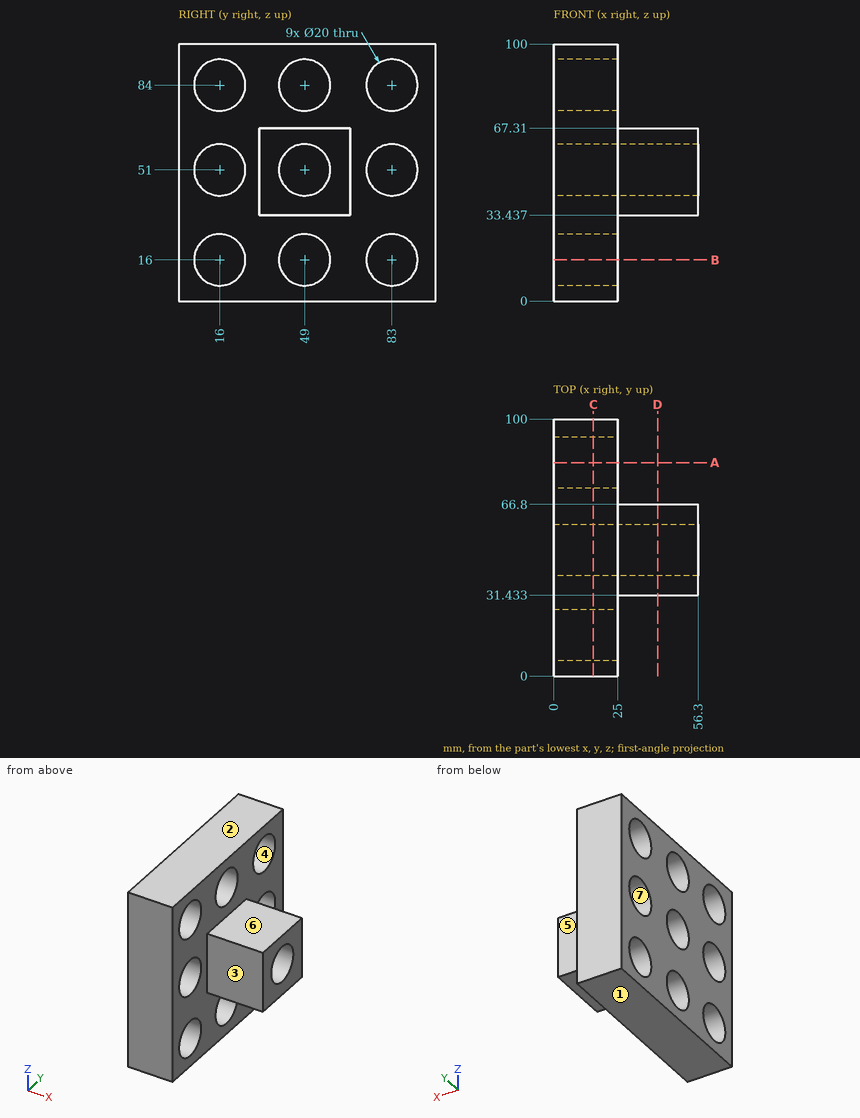
Study the drawing (mm; zero at the part's minimum x, y, z) and answer. A direction names the side the tool comes from. Give positions to 0.01 mm unless a question says otherwise; leave off trailing zeros. Loops run counter-clockwise (first coordinate to the right, second up) from the corner with the lowest first, then second, coordinate; pieces in that order, holes last. Notation, with made-up numbers: (3.5, -37) - (56.5, -37) arc R17 ccw to (56.5, -6) - close; hole circle Ø6 at (-31.5, 9.25). An arc over 180 degrees is marked (long way). One line per question, with ' | ' between items.
(1) The part is cut by section C-C (x = 15.5). Count the separate pieces of the cut face and the enclosed holes in it, then the cut area to 3 significant figures.
Recorded:
separate pieces: 1 | enclosed holes: 9 | area: 7,170 mm²
(2) A tool of negligible diameter and unlimited length cuts with its end or side. For the marked faces 5, 6 and 7, from which of +Z, -Z, +X, -X, +Y, -Y can it reach the whole face along a straight path? Write none if from no direction.
Recorded:
face 5: +Z, -Z, +X, +Y | face 6: +Z, +X, +Y, -Y | face 7: +X, -X
(3) Each of these flat-tipped pins is pushed along its axis until it touches: pin 1 Ø15.5 at (x, z) = (40, 57) entering from -Y; pin 2 Ø1.5 at (y, z) = (23.5, 81) entering from -X; pin 3 Ø9.5 at (x, y) = (46.5, 47.5) entering from -Z; pin 4 Ø4 at (y, z) = (77, 38.5) entering from +X. Where does it stop, or does it pass through?
Recorded:
pin 1: stops at y = 31.43 | pin 2: passes through | pin 3: stops at z = 33.44 | pin 4: stops at x = 25
(4) Straight lines are drawn through the part: probe 1 along Z at (x, y) = (17, 16); probe 2 along Z at (x, y) = (6, 90.5) (1 decimal); probe 3 along Y at (x, z) = (17, 80.5). For each, find the intervals that lie inside material, in ascending order.
Recorded:
probe 1: z = 0 to 6, 26 to 41, 61 to 74, 94 to 100 | probe 2: z = 0 to 9.4, 22.6 to 44.4, 57.6 to 77.4, 90.6 to 100 | probe 3: y = 0 to 6.63, 25.37 to 39.63, 58.37 to 73.63, 92.37 to 100
(5) The mould has two halves that part along Z. Classify the marked faces 1, 2, 3 and 4: +Z half, -Z half, draft (parallel to the pull), parting line (faces both ways), or undercut.
Recorded:
face 1: -Z half | face 2: +Z half | face 3: draft | face 4: undercut
(6) The part is cut by section B-B (z = 16). Write down the section's boundary in (x, y).
Recorded:
outline: (0, 0) - (25, 0) - (25, 6) - (0, 6) - close; (0, 26) - (25, 26) - (25, 39) - (0, 39) - close; (0, 59) - (25, 59) - (25, 73) - (0, 73) - close; (0, 93) - (25, 93) - (25, 100) - (0, 100) - close
(7) The part is cut by section D-D (x = 40.5). Write down the section's boundary in (y, z).
Recorded:
outline: (31.43, 33.44) - (66.8, 33.44) - (66.8, 67.31) - (31.43, 67.31) - close; hole circle Ø20 at (49, 51)
(8) The part is cut by section A-A (y = 83). Write down the section's boundary in (x, z), then the cut area to 3 significant figures.
Recorded:
outline: (0, 0) - (25, 0) - (25, 6) - (0, 6) - close; (0, 26) - (25, 26) - (25, 41) - (0, 41) - close; (0, 61) - (25, 61) - (25, 74) - (0, 74) - close; (0, 94) - (25, 94) - (25, 100) - (0, 100) - close | area: 1,000 mm²
